Autodesk Inventor part; units mm, degrees
ref_plane "YZ Plane" through (0, 0, 0) normal (1, 0, 0) x (0, 1, 0)
ref_plane "XZ Plane" through (0, 0, 0) normal (0, 1, 0) x (-1, 0, 0)
ref_plane "XY Plane" through (0, 0, 0) normal (0, 0, 1) x (1, 0, 0)
sketch "Эскиз1" plane through (0, 0, 0) normal (0, 0, 1) x (1, 0, 0)
  line L0 (5, 0) -> (92, 0)
  line L1 (97, 5) -> (97, 118)
  line L2 (92, 123) -> (5, 123)
  line L3 (0, 118) -> (0, 5)
  circle A0 centre (48.5, 48) radius 30
  arc A1 (5, 123) -> (0, 118) centre (5, 118) ccw
  arc A2 (97, 118) -> (92, 123) centre (92, 118) ccw
  arc A3 (92, 0) -> (97, 5) centre (92, 5) ccw
  arc A4 (0, 5) -> (5, 0) centre (5, 5) ccw
  arc A5 (46.5, 89) -> (50.5, 89) centre (48.5, 89) ccw
  arc A6 (50.5, 114) -> (46.5, 114) centre (48.5, 114) ccw
  line L4 (46.5, 89) -> (46.5, 114)
  line L5 (50.5, 114) -> (50.5, 89)
  circle A7 centre (48.5, 9.5) radius 2
  line L6 (12.1435, 79.8578) -> (12.1496, 83.1527)
  line L7 (12.1496, 83.1527) -> (15.0061, 84.7949)
  line L8 (15.0061, 84.7949) -> (17.8565, 83.1422)
  line L9 (17.8565, 83.1422) -> (17.8504, 79.8473)
  line L10 (17.8504, 79.8473) -> (14.9939, 78.2051)
  line L11 (14.9939, 78.2051) -> (12.1435, 79.8578)
  line L12 (12.1435, 12.8578) -> (12.1496, 16.1527)
  line L13 (12.1496, 16.1527) -> (15.0061, 17.7949)
  line L14 (15.0061, 17.7949) -> (17.8565, 16.1422)
  line L15 (17.8565, 16.1422) -> (17.8504, 12.8473)
  line L16 (17.8504, 12.8473) -> (14.9939, 11.2051)
  line L17 (14.9939, 11.2051) -> (12.1435, 12.8578)
  line L18 (79.1435, 12.8578) -> (79.1496, 16.1527)
  line L19 (79.1496, 16.1527) -> (82.0061, 17.7949)
  line L20 (82.0061, 17.7949) -> (84.8565, 16.1422)
  line L21 (84.8565, 16.1422) -> (84.8504, 12.8473)
  line L22 (84.8504, 12.8473) -> (81.9939, 11.2051)
  line L23 (81.9939, 11.2051) -> (79.1435, 12.8578)
  line L24 (79.1435, 79.8578) -> (79.1496, 83.1527)
  line L25 (79.1496, 83.1527) -> (82.0061, 84.7949)
  line L26 (82.0061, 84.7949) -> (84.8565, 83.1422)
  line L27 (84.8565, 83.1422) -> (84.8504, 79.8473)
  line L28 (84.8504, 79.8473) -> (81.9939, 78.2051)
  line L29 (81.9939, 78.2051) -> (79.1435, 79.8578)
  point P0 (0, 0)
  point P1 (97, 123)
  point P2 (0, 123)
  point P3 (15, 81.5)
  point P4 (15, 14.5)
  point P5 (15, 14.5)
  point P6 (82, 14.5)
  point P7 (82, 14.5)
  point P8 (82, 81.5)
  point P9 (82, 81.5)
  dimension "d10" = 5
  dimension "d21" = 4
  dimension "d22" = 4
  dimension "d23" = 4
extrude "Выдавливание1" add sketch "Эскиз1" along normal blind 4
properties part number "Адаптер для считывателя Bolid Proxy-2MA часть 2"
Read the model definition and answer for the solid it produces. Units are mm, in the model's axes. A direction names the side the tool comes from. Give positions to 0.01 mm unless a question says otherwise; leave off trailing zeros. Write each loop counter-clockwise with the first axis right and the second up, starting at its lowest first coordinate (ties: lowest second). Pieces come first, ordered by that corner, then holes. Notation, with made-up numbers: M -19,-7 L -13,-7 A26 cw -13,8 Z; hole C 65.5,86.5 d7. An arc over 180 degrees is marked long. Put each result on its own line as item: value. Start each with the question number.
1. Which of the six approach directions +Z, -Z, +X, -X, +Y, -Y give full straight-line access (tool end or side, diameter ignored) to faces 1 (the flat face through (80.59, 79.02, 1.97)), 2 (the flat face through (97, 61, 2))?
2. The part is cut by section A-A, the plane y = 9.5. Give the vertices of the cut face in (x, z), and give its area (3 significant figures).
3. Consider line 1 along Y through (x, z) = (48.5, 3); line 2 along X through (y, z) = (94.5, 1.5); line 3 along X through (y, z) = (83.5, 2.7). Determine where each line is inside the solid, lowest interval first.
4. The part is cut by section B-B, the plane x = 48.5. Give the vertices of the cut face in (y, z), and give its area (3 significant figures).
5. The part is cut by section C-C, the plane x = 59.5. Give the vertices of the cut face in (y, z).
6. The part is cut by section D-D, the plane z = 0.85. Give the number of separate pieces and of enclosed holes in the cut face, and give its area (3 significant figures).
7. For a pull along X with two mould halves and no side action, classify faces 3 (the cylindrical face through (48.5, 116, 2)), 4 (the flat face through (37, 76, 0)), 5 (the cylindrical face through (96, 2, 2)), 6 (the flat face through (83.41, 83.98, 1.97)) as released by +X, released by -X, zero draft, split by the parting line, or undercut.
Final values:
1. face 1: +Z, -Z
1. face 2: +Z, -Z, +X, +Y, -Y
2. outline: M 0,0 L 46.5,0 L 46.5,4 L 0,4 Z; M 50.5,0 L 97,0 L 97,4 L 50.5,4 Z
2. area: 372 mm²
3. line 1: y = 0 to 7.5, 11.5 to 18, 78 to 87, 116 to 123
3. line 2: x = 0 to 46.5, 50.5 to 97
3. line 3: x = 0 to 12.75, 17.24 to 79.75, 84.24 to 97
4. outline: M 0,0 L 7.5,0 L 7.5,4 L 0,4 Z; M 11.5,0 L 18,0 L 18,4 L 11.5,4 Z; M 78,0 L 87,0 L 87,4 L 78,4 Z; M 116,0 L 123,0 L 123,4 L 116,4 Z
4. area: 120 mm²
5. outline: M 0,0 L 20.09,0 L 20.09,4 L 0,4 Z; M 75.91,0 L 123,0 L 123,4 L 75.91,4 Z
6. separate pieces: 1
6. enclosed holes: 7
6. area: 8,840 mm²
7. face 3: undercut
7. face 4: zero draft
7. face 5: released by +X
7. face 6: undercut
